Part model, mm, in its own coordinate system. Give positions to 0.01 mm unless a question says otherwise; leave off trailing zeros. Write each loop counter-clockwise with the first axis right and the second up, starting at its lowest first coordinate (ties: lowest second). Pieces come first, ordered by that corner, then holes.
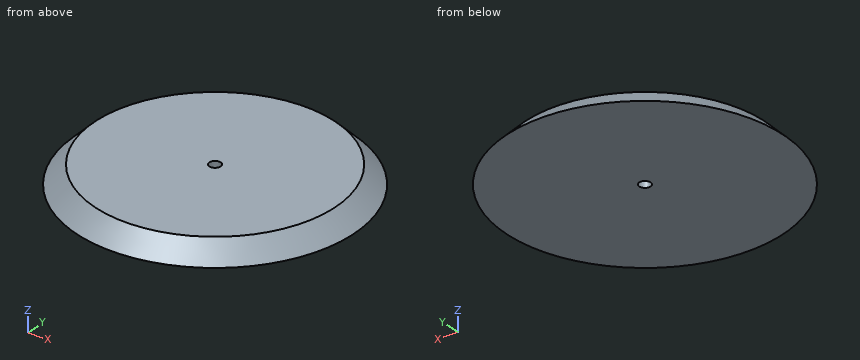
from build123d import *

# Parameters (mm, degrees)
F0_R     = 31.75
F1_DEPTH = 4.1021592915
F5_D     = 2.54


# Not quite as in the source:
# - a fillet or chamfer that OpenCascade refuses, or shapes differently, is made with other operations: its cross-section is extruded or revolved along the edge and cut away or added
# - the program builds the solid bodies; features that only make, move or delete a surface that nothing else refers to are left out


with BuildPart() as f1:
    # F0 (on Top) → F1 (new body)
    with BuildSketch(Plane.XY):
        Circle(F0_R)
    extrude(amount=F1_DEPTH)

    # F2: chamfer of 5.08 on 1 edges, made by hand

    # F2_s1 → F2_t2 (revolve, cut)
    with BuildSketch(Plane.XZ):
        Polygon((31.75, -0.9778407085), (26.67, 4.1021592915), (31.75, 4.1021592915), align=None)
    revolve(axis=Axis((0, 0, 4.1021592915), (0, 0, 1)), mode=Mode.SUBTRACT)

    # F5 (through all)
    with Locations(Plane.XY.offset(4.1021592915)):
        with Locations((0, 0)):
            Hole(F5_D / 2)


solid = f1.part
1) Drill centre lines: L1, parallel to X at y = 9, z = 0.7; L2, parallel to Y at x = 0, z = 1.25; L3, parallel to Y at x = 12, z = 3.2. Where is each one in solid material? Low to high.
Check result:
L1: x = -28.69 to 28.69
L2: y = -29.52 to -1.27, 1.27 to 29.52
L3: y = -24.82 to 24.82
2) Saw through at C-C (z = 1.05). Write the cut outline in (x, y).
Check result:
outline: circle Ø59.44 at (0, 0); hole circle Ø2.54 at (0, 0)
3) Saw through at A-A (y = 0). Write the cut outline in (x, z), and give its area (3 significant figures).
Check result:
outline: (-30.77, 0) - (-1.27, 0) - (-1.27, 4.1) - (-26.67, 4.1) - close; (1.27, 0) - (30.77, 0) - (26.67, 4.1) - (1.27, 4.1) - close
area: 225 mm2
